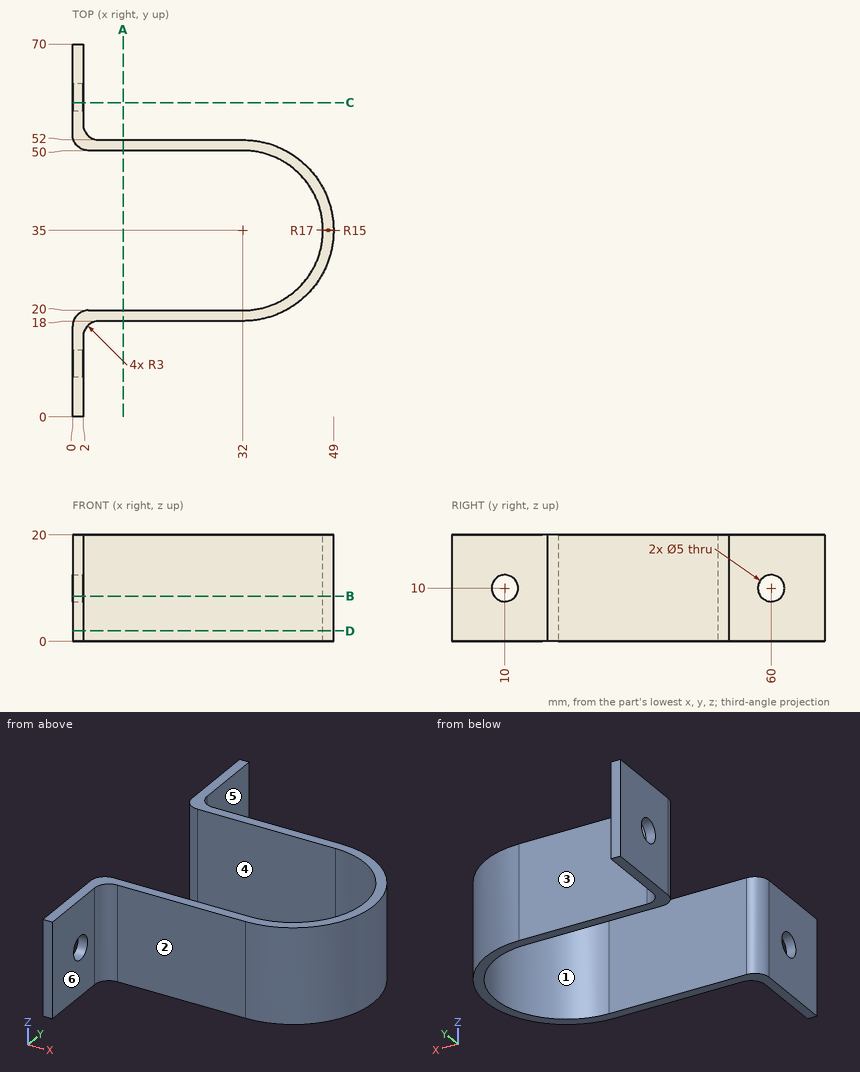
Geometry: see drawing. Coordinates: mm, zero at the bounding-box minimum. A direction names the side the tool comes from. Coordinates: 2 decimals unless noted, no trailing zeros. Loops run counter-clockwise (first coordinate to the right, second up) from the corner with the lowest first, then second, coordinate; pieces in that order, holes last.
(1) Section D-D on z = 2. Return the cut outline in (x, y).
(2) Set-up query: the marked faces 4, 5 and 6. Return all of +Z, -Z, +X, -X, +Y, -Y with unobstructed straight access to the full face (end or side cutting, diameter ignored); none if empty.
(3) Section A-A on x = 9.5. Return the cut outline in (y, z).
(4) Section B-B on z = 8.5. Return the cut outline in (x, y).
(5) Pull-direction query (Y, two-part tool) for the marked faces 1, 2 and 3; classes: released by +Y, released by -Y, zero draft, split by the parting line, or undercut.
(6) Material intervals for probe 1 along Z at (x, y) = (0.5, 10); probe 2 along Y at (x, z) = (25.5, 17.75); probe 3 along X at (y, z) = (10.5, 6.5), sorted ascending.
(7) First-contact query: pin 1 Ø4.5 at (y, z) = (61, 8.5) entering from +X; pin 2 Ø10 at (x, z) = (22.5, 14.5) entering from -Y; pin 3 Ø1.5 at (x, y) = (19.5, 18.5) entering from -Z; pin 4 Ø4 at (y, z) = (60, 10) entering from +X. Flat tips, straight axial feed; report the tip coordinate or a pass-through.
(8) Section C-C on y = 59. Return the cut outline in (x, z).
Data:
1. outline: (0, 0) - (2, 0) - (2, 15) arc R3 cw to (5, 18) - (32, 18) arc R17 ccw to (32, 52) - (5, 52) arc R3 cw to (2, 55) - (2, 70) - (0, 70) - (0, 53) arc R3 ccw to (3, 50) - (32, 50) arc R15 cw to (32, 20) - (3, 20) arc R3 ccw to (0, 17) - close
2. face 4: +Z, -Z, -X
2. face 5: +Z, -Z, +X, +Y
2. face 6: +Z, -Z, +X, -Y
3. outline: (18, 0) - (20, 0) - (20, 20) - (18, 20) - close; (50, 0) - (52, 0) - (52, 20) - (50, 20) - close
4. outline: (0, 0) - (2, 0) - (2, 8) - (0, 8) - close; (0, 12) - (2, 12) - (2, 15) arc R3 cw to (5, 18) - (32, 18) arc R17 ccw to (32, 52) - (5, 52) arc R3 cw to (2, 55) - (2, 58) - (0, 58) - (0, 53) arc R3 ccw to (3, 50) - (32, 50) arc R15 cw to (32, 20) - (3, 20) arc R3 ccw to (0, 17) - close; (0, 62) - (2, 62) - (2, 70) - (0, 70) - close
5. face 1: undercut
5. face 2: released by -Y
5. face 3: released by +Y
6. probe 1: z = 0 to 7.5, 12.5 to 20
6. probe 2: y = 18 to 20, 50 to 52
6. probe 3: x = 0 to 2
7. pin 1: stops at x = 2
7. pin 2: stops at y = 18
7. pin 3: stops at z = 0
7. pin 4: passes through
8. outline: (0, 0) - (2, 0) - (2, 7.71) - (0, 7.71) - close; (0, 12.29) - (2, 12.29) - (2, 20) - (0, 20) - close
